from build123d import *

# Parameters (mm, degrees)
F1_DEPTH   = 25.4
F1_FACE_W  = 25.4
F1_FACE_H  = 44.3220827729
F1_FACE1_W = 30.3635057062
F1_FACE1_H = 17.8439561278


with BuildPart() as f1:
    # F0 (on Front) → F1 (new body)
    with BuildSketch(Plane.XZ):
        Polygon((0, 54.8269934952), (-24.0317806602, 28.3488668501), (0, 28.3488668501), align=None)
        Polygon((0, 28.3488668501), (-24.0317806602, 28.3488668501), (-24.0317806602, -12.5195495784), (0, 10.5049107224), align=None)
        Polygon((0, 54.8269934952), (0, 28.3488668501), (30.3635057062, 28.3488668501), (53.6757707596, 54.8269934952), align=None)
        Polygon((0, 10.5049107224), (-24.0317806602, -12.5195495784), (30.3635057062, -12.5195495784), (30.3635057062, 10.5049107224), align=None)
        Polygon((53.6757707596, 54.8269934952), (30.3635057062, 28.3488668501), (30.3635057062, 10.5049107224), (53.6757707596, 10.5049107224), align=None)
        Polygon((30.3635057062, 10.5049107224), (30.3635057062, -12.5195495784), (53.6757707596, 10.5049107224), align=None)
    extrude(amount=F1_DEPTH)

    # F1_face (on face) + F1_face1 (on face) → F2 (revolve)
    with BuildSketch(Plane(origin=(53.6757707596, -12.7, 32.6659521088), x_dir=(0, 1, 0), z_dir=(1, 0, 0))):
        Rectangle(F1_FACE_W, F1_FACE_H)
    with BuildSketch(Plane(origin=(15.1328731022, -25.4, 21.1555782678), x_dir=(1, 0, 0), z_dir=(0, -1, 0))):
        Polygon((-39.1646537623, -33.6751278462), (15.230632604, -33.6751278462), (38.5428976574, -10.6506675454), (38.5428976574, 33.6714152274), (-15.1328731022, 33.6714152274), (-39.1646537623, 7.1932885823), align=None)
        with Locations((0.0488797509, -1.7286894816)):
            Rectangle(F1_FACE1_W, F1_FACE1_H, mode=Mode.SUBTRACT)
    revolve(axis=Axis((53.6757707596, -25.4, 32.6659521088), (0, 0, 1)))


solid = f1.part
Could you check a few things on this model? Use its own coordinates, in mm. A direction names the side the tool comes from. Round coordinates to 2 decimals unless told otherwise and drop trailing zeros. Loops run counter-clockwise (first coordinate to the right, second up) from the corner with the lowest first, then second, coordinate; pieces in that order, holes last. Notation, with made-up numbers: (55.5, 26) -> (66.5, 26) arc R24 cw to (66.5, 37) -> close; hole circle Ø9 at (64.5, 71.5). An arc over 180 degrees is marked (long way). Use CSV: the item, a comma, the result in double quotes.
(1) Will these pins go through, and if not, where does the flat tip stop? pin 1 Ø2 at (y, z) = (-37.5, 11) entering from +X; pin 2 Ø4 at (x, z) = (20.5, -1.5) entering from -Y; pin 3 Ø1.5 at (x, z) = (16.5, 38.5) entering from +Y; pin 4 Ø6 at (x, y) = (68, -80) entering from +Z.
Return value:
pin 1,"stops at x = 130.59"
pin 2,"stops at y = -96.58"
pin 3,"stops at y = 33.07"
pin 4,"stops at z = 54.83"
(2) For faces 1 (the flat face through (42, 0, 20)), 2 (the flat face through (-11.85, -12.52, 41.77)), 3 (the flat face through (-20, 0, 21)), which set-ups out of +Z, -Z, +X, -X, +Y, -Y let a thin tool reach every point of the face, with its end or its side?
Return value:
face 1,"none"
face 2,"+Z, -X, +Y, -Y"
face 3,"+Z, -X, +Y"
(3) If I drill on probe 1 along X at (y, z) = (-25, 19); probe 2 along Z at (x, y) = (91, -54); probe 3 along Y at (x, z) = (65, -4), over which ranges is the centre line in solid material (lowest first)? Write a range as [from, to].
Return value:
probe 1,"x = [-24.03, 0], [28.28, 79.07], [107.35, 131.38]"
probe 2,"z = [-12.52, 10.5], [28.35, 54.83]"
probe 3,"y = [-102.28, -34.75], [-16.05, 51.48]"
(4) Suppose I cut it at D-D on z = 43.5. Write out the boundary of the cut face in (x, y).
Return value:
outline,"(-10.28, -25.4) arc R63.96 ccw (long way) to (-5.02, 0) -> (-10.28, 0) -> close"
(5) If we mould it in two halves opening along Y, with no side actions, what happens to faces 4 (the conical face through (107.664, -36.802, 53.171)), 5 (the flat face through (65, -49, 28.349)), 6 (the flat face through (-24.032, -13, 8))? For each: +Y half, -Y half, draft (parallel to the pull), parting line (faces both ways), or undercut.
Return value:
face 4,"parting line"
face 5,"undercut"
face 6,"draft"
(6) Suppose I cut it at B-B on x = 59.5. Give the number of separate pieces and of enclosed holes in the cut face, plus the area to 3 significant figures.
Return value:
separate pieces,"1"
enclosed holes,"2"
area,"8,330 mm²"
(7) Suppose I cut it at A-A on z = 21. Write out the boundary of the cut face in (x, y).
Return value:
outline,"(-24.03, -25.4) arc R77.71 ccw (long way) to (-19.76, 0) -> (-24.03, 0) -> close; (30.36, -15.32) arc R25.4 ccw (long way) to (53.68, 0) -> (30.36, 0) -> close; hole circle Ø107.35 at (53.68, -25.4)"
